Geometry: final body of the model. Coordinates: model frame, mm. A direction names the side the tool comes from. Coordinates: 2 decimals unless noted, no trailing zeros. Loops run counter-clockwise (first coordinate to the right, second up) from the corner with the lowest first, then second, coordinate; pieces in that order, holes last. Notation, with made-up numbers: (39.25, 55.25) - (56.25, 55.25) arc R19 ccw to (56.25, 71.25) - close; hole circle Ø5 at (82.5, 37). An arc over 180 degrees is marked (long way). Answer in a Markdown table with one row per item.
from build123d import *

# Parameters (mm, degrees)
BOSS_EXTRUDE1_DEPTH = 5
SKETCH2_R           = 4.25
SKETCH2_R_2         = 1
SKETCH2_W           = 5
SKETCH2_H           = 6
SKETCH2_W_2         = 24
SKETCH2_H_2         = 5
CUT_EXTRUDE1_DEPTH  = 5


with BuildPart() as part:
    # Sketch1 → Boss-Extrude1 (new body)
    with BuildSketch(Plane(origin=(0, 0, 0), x_dir=(1, 0, 0), z_dir=(0, 1, 0))):
        Polygon((-16, -42.5), (16, -42.5), (16, -2.5), (30, 0), (30, 20), (16, 22.5), (16, 42.5), (-16, 42.5), (-16, 22.5), (-30, 20), (-30, 0), (-16, -2.5), align=None)
    extrude(amount=BOSS_EXTRUDE1_DEPTH)

    # Sketch2 → Cut-Extrude1 (cut)
    with BuildSketch(Plane(origin=(0, 5, 0), x_dir=(1, 0, 0), z_dir=(0, 1, 0))):
        with Locations(Location((0, -27.5, 0), (0, 0, 270))):
            Circle(SKETCH2_R)
        with Locations(Location((-8, -27.5, 0), (0, 0, 270))):
            Circle(SKETCH2_R_2)
        with Locations(Location((0, -19.5, 0), (0, 0, 270))):
            Circle(SKETCH2_R_2)
        with Locations(Location((8, -27.5, 0), (0, 0, 270))):
            Circle(SKETCH2_R_2)
        with Locations(Location((0, -35.5, 0), (0, 0, 270))):
            Circle(SKETCH2_R_2)
        with Locations((-26, 10)):
            Rectangle(SKETCH2_W, SKETCH2_H)
        with Locations((26, 10)):
            Rectangle(SKETCH2_W, SKETCH2_H)
        with Locations((0, 30)):
            Rectangle(SKETCH2_W_2, SKETCH2_H_2)
    extrude(amount=-CUT_EXTRUDE1_DEPTH, mode=Mode.SUBTRACT)


solid = part.part
(1) Cut plane C-C on x = 0. Output: boundary loops of the cut face in (y, z).
Verdict:
| item | result |
|---|---|
| outline | (0, -42.5) - (5, -42.5) - (5, -32.5) - (0, -32.5) - close; (0, -27.5) - (5, -27.5) - (5, 18.5) - (0, 18.5) - close; (0, 20.5) - (5, 20.5) - (5, 23.25) - (0, 23.25) - close; (0, 31.75) - (5, 31.75) - (5, 34.5) - (0, 34.5) - close; (0, 36.5) - (5, 36.5) - (5, 42.5) - (0, 42.5) - close |
(2) Pull-direction query (X, two-part tool) for faces 4 (the face through (16, 2, -32)), 5 (the face through (-28.5, 3, -10)), 6 (the face through (-26, 3, -7)), 7 (the face through (0, 5, -1)); classes: pulls with the +X half, pulls with the -X half, needs draft (parallel to the pull), parting line crosses it, or undercut.
Verdict:
| item | result |
|---|---|
| face 4 | pulls with the +X half |
| face 5 | undercut |
| face 6 | undercut |
| face 7 | needs draft |
(3) Cut plane A-A on x = -8. Output: boundary loops of the cut face in (y, z), then the cut area to 3 significant figures.
Verdict:
| item | result |
|---|---|
| outline | (0, -42.5) - (5, -42.5) - (5, -32.5) - (0, -32.5) - close; (0, -27.5) - (5, -27.5) - (5, 26.5) - (0, 26.5) - close; (0, 28.5) - (5, 28.5) - (5, 42.5) - (0, 42.5) - close |
| area | 390 mm² |
(4) Ray query, probe 1 along X at (y, z) = (1.75, 27.5); probe 2 along Z at (x, y) = (-5, 3); probe 3 along X at (y, z) = (2.65, 35.5). Return the intervals inside material, ascending.
Verdict:
| item | result |
|---|---|
| probe 1 | x = -16 to -9, -7 to -4.25, 4.25 to 7, 9 to 16 |
| probe 2 | z = -42.5 to -32.5, -27.5 to 42.5 |
| probe 3 | x = -16 to -1, 1 to 16 |
(5) First-contact query: pin 1 Ø1.5 at (x, z) = (-0.5, 24.5) entering from +Y; pin 2 Ø2.5 at (x, y) = (26, 2) entering from -Z; pin 3 Ø2.5 at (x, y) = (26, 3.5) entering from +Z; pin 4 Ø4 at (x, z) = (18, -11) entering from -Y. Flat tips, straight axial feed; report the tip coordinate or a pass-through.
Verdict:
| item | result |
|---|---|
| pin 1 | passes through |
| pin 2 | stops at z = -20.94 |
| pin 3 | stops at z = 0.94 |
| pin 4 | stops at y = 0 |
(6) Cut plane D-D on y = 4.15. State how many separate pieces and enclosed holes the cut face has, then the cut area to 3 significant figures.
Verdict:
| item | result |
|---|---|
| separate pieces | 1 |
| enclosed holes | 8 |
| area | 3,100 mm² |
(7) Cut plane B-B on z = 35.5. Output: boundary loops of the cut face in (x, y), then the cut area to 3 significant figures.
Verdict:
| item | result |
|---|---|
| outline | (-16, 0) - (-1, 0) - (-1, 5) - (-16, 5) - close; (1, 0) - (16, 0) - (16, 5) - (1, 5) - close |
| area | 150 mm² |
(8) Access query for faces 1 (the face through (-23.098, 2.465, 1.233)), 2 (the face through (16, 2, 23)), 3 (the face through (-23.5, 3, -10)). Directions: +Z, -Z, +X, -X, +Y, -Y. A direction counts if a zero-diameter tool reaches every point of the face in a straight line with its end or side. Return the directions, or none.
Verdict:
| item | result |
|---|---|
| face 1 | +Z, -X, +Y, -Y |
| face 2 | +Z, +X, +Y, -Y |
| face 3 | +Y, -Y |
